Work out the finished part from the listing and answer in its coordinate system (mm). A direction names the side the tool comes from. Round coordinates to 2 decimals unless told otherwise and drop trailing zeros. Write each loop counter-clockwise with the first axis right and the second up, starting at its lowest first coordinate (ties: lowest second). Pieces come first, ordered by that corner, then holes. Notation, with made-up numbers: (-7.75, 82.5) -> (26.25, 82.5) arc R17 ccw to (26.25, 112.5) -> close; hole circle Ø8 at (18.25, 2.25). An arc over 180 degrees is marked (long way). Answer as a JSON object with one key per item and string values. Group by question number.
from build123d import *

# Parameters (mm, degrees)
F0_R     = 8.5
F1_DEPTH = 15
F2_R     = 10
F3_DEPTH = 5


# Not quite as in the source:
# - a fillet or chamfer that OpenCascade refuses, or shapes differently, is made with other operations: its cross-section is extruded or revolved along the edge and cut away or added


with BuildPart() as f1:
    # F0 (on Front) → F1 (new body)
    with BuildSketch(Plane.XZ):
        Circle(F0_R)
    extrude(amount=F1_DEPTH)

    # F2 (on face) → F3 (join)
    with BuildSketch(Plane.XZ.offset(15)):
        Circle(F2_R)
    extrude(amount=F3_DEPTH)

    # F4: fillet of radius 9.8982756057 on 1 edges, made by hand

    # F4_s1 → F4_t2 (revolve, cut)
    with BuildSketch(Plane.XY):
        with BuildLine():
            ThreePointArc((10, -15), (6.3731809715, -18.6591872749), (1.3986770752, -20))
            Line((1.3986770752, -20), (10, -20))
            Line((10, -20), (10, -15))
        make_face()
    revolve(axis=Axis((0, -20, 0), (0, -1, 0)), mode=Mode.SUBTRACT)


solid = f1.part
1) Each of these flat-tipped pins is pushed along its axis until it touches: P1, Ø10, axis at x = 4.5, y = -4.5, coming from the +Z side; P2, Ø1, axis at x = 1, y = -12.5, coming from the -Z side; P3, Ø1, axis at x = 2, z = 1, coming from the -Y side. Where does it stop, or does it pass through?
2) A cutting plane is placed at A-A on y = -5.5. Determine the outline of the cut face in (x, z), plus the area to 3 significant figures.
3) A tool of negligible diameter and unlimited length cuts with its end or side. For faces 1 (the face through (4.57, -7.395, 7.167)), 2 (the face through (0, -20, 0)), from which of +Z, -Z, +X, -X, +Y, -Y can it reach the whole face along a straight path? Write none if from no direction.
4) Straight lines are drawn through the part: L1, parallel to Z at x = 0.25, y = -14; L2, parallel to X at y = -10.25, z = 4.5; L3, parallel to Y at x = 5.75, z = -7.75. For each, find the intervals that lie inside material, in ascending order.
Established:
{
 "1": {"P1": "stops at z = 8.5", "P2": "stops at z = -8.49", "P3": "stops at y = -19.99"},
 "2": {"outline": "circle Ø17 at (0, 0)", "area": "227 mm²"},
 "3": {"face 1": "+Y", "face 2": "+Z, -Z, +X, -X, -Y"},
 "4": {"L1": "z = -8.5 to 8.5", "L2": "x = -7.21 to 7.21", "L3": "y = -15.57 to -15"}
}
